Input: part model. Units: mm. Frame: model coordinates. Face numbers are marked on the shaded views. A direction names the side the tool comes from. Give positions to 0.01 mm unless a question says otherwise; leave off trailing zeros. Order: outer loops, then holes, each group sorted by start corner. A loop starts at its lowest first (then second) coordinate and runs counter-clockwise, first axis right, second up. Notation, with made-up numbers: (-12, -12.75) - (16, -12.75) arc R22 cw to (16, 21.25) - close; hole circle Ø7 at (-25, -27). An arc over 180 degrees is marked (long way). Use a Markdown table: item, result.
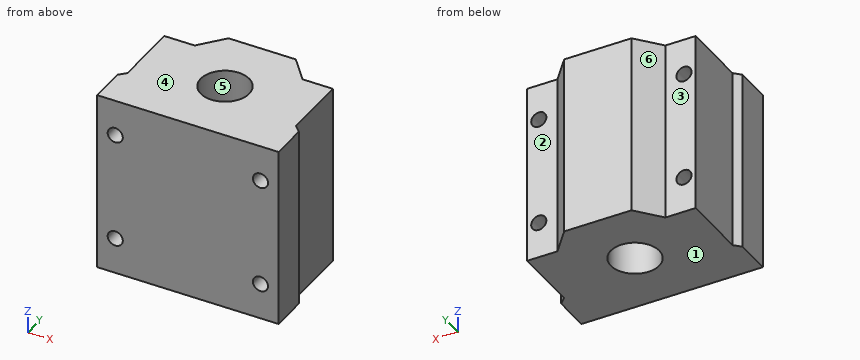
from build123d import *

# Parameters (mm, degrees)
SKETCH1_R             = 4
BOSS_EXTRUDE1_DEPTH   = 30
F_2_5MM_DOWEL_HOLE1_D = 2.5


with BuildPart() as part:
    # Sketch1 → Boss-Extrude1 (new body)
    with BuildSketch(Plane.XY):
        Polygon((-15, -11), (15, -11), (15, -5), (13.93169164, -3.93169164), (13.93169164, 7), (8.917679795, 7), (5.56128127, 11), (-5.56128127, 11), (-8.917679795, 7), (-13.93169164, 7), (-13.93169164, -3.93169164), (-15, -5), align=None)
        Circle(SKETCH1_R, mode=Mode.SUBTRACT)
    extrude(amount=-BOSS_EXTRUDE1_DEPTH)

    # Ø2.5mm Dowel Hole1 (through all)
    with Locations(Plane(origin=(0, 7, 0), x_dir=(1, 0, 0), z_dir=(0, 1, 0))):
        with Locations((-12, 24), (-12, 6), (12, 6), (12, 24)):
            Hole(F_2_5MM_DOWEL_HOLE1_D / 2)


solid = part.part
1. Set-up query: the marked faces 1, 2 and 3. Return all of +Z, -Z, +X, -X, +Y, -Y with unobstructed straight access to the full face (end or side cutting, diameter ignored); none if empty.
Response:
| item | result |
|---|---|
| face 1 | -Z, +X, -X, +Y, -Y |
| face 2 | +Z, -Z, +X, +Y |
| face 3 | +Z, -Z, -X, +Y |
2. Material intervals for line 1 along Z through (x, y) = (-12, 0); line 2 along X through (y, z) = (-3.5, -6); line 3 along X through (y, z) = (-0.75, -6), sorted ascending.
Response:
| item | result |
|---|---|
| line 1 | z = -30 to -25.25, -22.75 to -7.25, -4.75 to 0 |
| line 2 | x = -13.93 to -13.25, -10.75 to -1.94, 1.94 to 10.75, 13.25 to 13.93 |
| line 3 | x = -13.93 to -13.25, -10.75 to -3.93, 3.93 to 10.75, 13.25 to 13.93 |
3. Section query A-A (z = -5.25). Return loops of the section in (x, y), then the cut area to 3 significant figures.
Response:
| item | result |
|---|---|
| outline | (-15, -11) - (-13, -11) - (-13, 7) - (-13.93, 7) - (-13.93, -3.93) - (-15, -5) - close; (-11, -11) - (11, -11) - (11, 7) - (8.92, 7) - (5.56, 11) - (-5.56, 11) - (-8.92, 7) - (-11, 7) - close; (13, -11) - (15, -11) - (15, -5) - (13.93, -3.93) - (13.93, 7) - (13, 7) - close; hole circle Ø8 at (0, 0) |
| area | 451 mm^2 |
4. Section query B-B (x = -12). Return loops of the section in (y, z).
Response:
| item | result |
|---|---|
| outline | (-11, -30) - (7, -30) - (7, -25.25) - (-11, -25.25) - close; (-11, -22.75) - (7, -22.75) - (7, -7.25) - (-11, -7.25) - close; (-11, -4.75) - (7, -4.75) - (7, 0) - (-11, 0) - close |
5. Pin query (flat end, axial travel): pin 1 (2 mm diameter, centred on x = 12, z = -24, fed in from -Y); pin 2 (8.5 mm diameter, centred on y = -0.5, z = -16.5, fed in from +X); pin 3 (3 mm diameter, centred on x = 12, z = -6, fed in from +Y); pin 4 (10 mm diameter, centred on y = 7.5, z = -11, fed in from +X). Return the tip coordinate at first contact, or that it passes through.
Response:
| item | result |
|---|---|
| pin 1 | passes through |
| pin 2 | stops at x = 14.75 |
| pin 3 | stops at y = 7 |
| pin 4 | stops at x = 13.93 |
6. Section query C-C (y = -3.5). Return loops of the section in (x, z).
Response:
| item | result |
|---|---|
| outline | (-13.93, -30) - (-1.94, -30) - (-1.94, 0) - (-13.93, 0) - close; (1.94, -30) - (13.93, -30) - (13.93, 0) - (1.94, 0) - close; hole circle Ø2.5 at (-12, -24); hole circle Ø2.5 at (-12, -6); hole circle Ø2.5 at (12, -24); hole circle Ø2.5 at (12, -6) |
7. Section query D-D (z = -10). Return loops of the section in (x, y), then the cut area to 3 significant figures.
Response:
| item | result |
|---|---|
| outline | (-15, -11) - (15, -11) - (15, -5) - (13.93, -3.93) - (13.93, 7) - (8.92, 7) - (5.56, 11) - (-5.56, 11) - (-8.92, 7) - (-13.93, 7) - (-13.93, -3.93) - (-15, -5) - close; hole circle Ø8 at (0, 0) |
| area | 523 mm^2 |
8. Mould query, pull axis X, two halves, no side actions, for the marked faces 4, 5 and 6. Classes: pulls with the +X half, pulls with the -X half, needs draft (parallel to the pull), parting line crosses it, or undercut.
Response:
| item | result |
|---|---|
| face 4 | needs draft |
| face 5 | undercut |
| face 6 | pulls with the -X half |
